```python
from build123d import *

# Parameters (mm, degrees)
F1_DEPTH = 12.7
F2_R     = 5.08
F3_R     = 5.08


with BuildPart() as f1:
    # F0 (on Front) → F1 (new body)
    with BuildSketch(Plane.XZ):
        with BuildLine():
            ThreePointArc((71.501, 44.45), (19.90199, 65.82301), (41.275, 14.224))
            ThreePointArc((41.275, 14.224), (62.64801, 23.07699), (71.501, 44.45))
        make_face()
        with BuildLine():
            ThreePointArc((71.5391, 361.95), (62.67495, 383.34995), (41.275, 392.2141))
            ThreePointArc((41.275, 392.2141), (19.87505, 340.55005), (71.5391, 361.95))
        make_face()
        Polygon((0, 406.4), (0, 0), (41.275, 0), (82.55, 0), (82.55, 406.4), (41.275, 406.4), align=None)
        with BuildLine():
            ThreePointArc((71.501, 44.45), (62.64801, 23.07699), (41.275, 14.224))
            ThreePointArc((41.275, 14.224), (19.90199, 65.82301), (71.501, 44.45))
        make_face(mode=Mode.SUBTRACT)
        with BuildLine():
            ThreePointArc((71.5391, 361.95), (19.87505, 340.55005), (41.275, 392.2141))
            ThreePointArc((41.275, 392.2141), (62.67495, 383.34995), (71.5391, 361.95))
        make_face(mode=Mode.SUBTRACT)
    extrude(amount=F1_DEPTH)

    # F2
    f2_edges = [f1.edges().sort_by_distance(p)[0] for p in [
        (82.55, -6.35, 406.4),
    ]]
    fillet(f2_edges, radius=F2_R)

    # F3
    f3_edges = [f1.edges().sort_by_distance(p)[0] for p in [
        (0, -6.35, 406.4),
        (82.55, -6.35, 0),
        (0, -6.35, 0),
    ]]
    fillet(f3_edges, radius=F3_R)


solid = f1.part
```
Geometry: final body of the model. Coordinates: model frame, mm. Round coordinates to 2 decimals unless told otherwise and drop trailing zeros. Loops run counter-clockwise (first coordinate to the right, second up) from the corner with the lowest first, then second, coordinate; pieces in that order, holes last. Notation, with made-up numbers: (25, -8.75) -> (32, -8.75) arc R18 ccw to (32, 21.25) -> close; hole circle Ø6 at (-24, 14.25). An arc over 180 degrees is marked (long way). Write each question's results on one line, items separated by ' | '.
Item 1: Cut plane C-C on z = 38.5. Return the cut outline in (x, y), and give its area (3 significant figures).
Answers below:
outline: (0, -12.7) -> (11.64, -12.7) -> (11.64, 0) -> (0, 0) -> close; (70.91, -12.7) -> (82.55, -12.7) -> (82.55, 0) -> (70.91, 0) -> close | area: 296 mm²
Item 2: Cut plane A-A on y = -6. Return the cut outline in (x, z) (3 decimals).
Answers below:
outline: (0, 5.08) arc R5.08 ccw to (5.08, 0) -> (77.47, 0) arc R5.08 ccw to (82.55, 5.08) -> (82.55, 401.32) arc R5.08 ccw to (77.47, 406.4) -> (5.08, 406.4) arc R5.08 ccw to (0, 401.32) -> close; hole (41.275, 14.224) arc R30.226 ccw to (71.501, 44.45) arc R30.226 ccw (long way) to start; hole (41.275, 392.214) arc R30.264 ccw (long way) to (71.539, 361.95) arc R30.264 ccw to start
Item 3: Cut plane D-D on x = 16.5. Return the cut outline in (y, z), and give its area (3 significant figures).
Answers below:
outline: (-12.7, 0) -> (0, 0) -> (0, 27.13) -> (-12.7, 27.13) -> close; (-12.7, 61.77) -> (0, 61.77) -> (0, 344.57) -> (-12.7, 344.57) -> close; (-12.7, 379.33) -> (0, 379.33) -> (0, 406.4) -> (-12.7, 406.4) -> close | area: 4,280 mm²
Item 4: Cut plane B-B on x = 50.5. Return the cut outline in (y, z), and give its area (3 significant figures).
Answers below:
outline: (-12.7, 0) -> (0, 0) -> (0, 15.67) -> (-12.7, 15.67) -> close; (-12.7, 73.23) -> (0, 73.23) -> (0, 333.13) -> (-12.7, 333.13) -> close; (-12.7, 390.77) -> (0, 390.77) -> (0, 406.4) -> (-12.7, 406.4) -> close | area: 3,700 mm²
Item 5: Line query: probe 1 along Z at (x, y) = (18.5, -11); probe 2 along Z at (x, y) = (21, -2.25); probe 3 along X at (y, z) = (-6, 361.95). Output: solid intervals per line, ascending. Write a range as [from, to].
Answers below:
probe 1: z = [0, 24.58], [64.32, 342.02], [381.88, 406.4] | probe 2: z = [0, 22.03], [66.87, 339.48], [384.42, 406.4] | probe 3: x = [0, 11.01], [71.54, 82.55]
